Input: part model. Units: mm. Frame: model coordinates. Round coordinates to 2 decimals unless told otherwise and drop trailing zeros. Write each loop counter-clockwise with the first axis right and the second up, starting at its lowest first coordinate (ties: lowest second). Pieces come first, ordered by that corner, then holes. Notation, with made-up numbers: M -28,21 L 26,21 A20 ccw 26,28 Z; hole C 27,43 d11. An arc over 180 degrees is marked long. Answer as CSV lines item,"result". Start each with the question number.
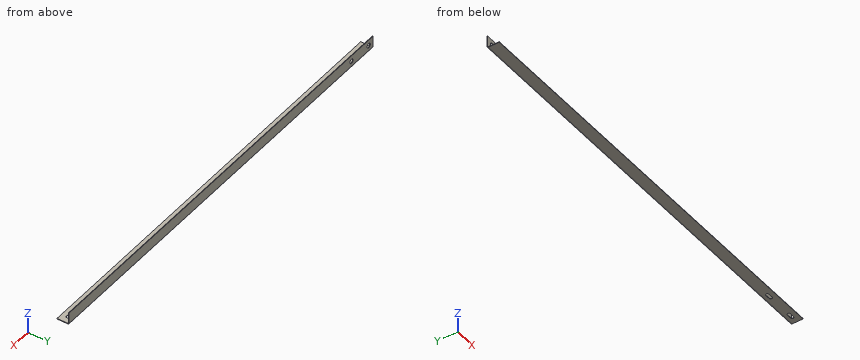
```python
from build123d import *

# Parameters (mm, degrees)
SKETCH1_W                    = 1415
SKETCH1_H                    = 40
BASE_FLANGE1_DEPTH           = 2
EDGE_FLANGE1_STRIP_W         = 13
EDGE_FLANGE1_STRIP_H         = 2
EDGE_FLANGE1_STRIP_CUT_DEPTH = 1415
EDGE_FLANGE1_DEPTH           = 1415
SKETCH9_R                    = 7.5
CUT_EXTRUDE1_DEPTH           = 920.516022359


# Sheet-metal steps are written as plain solids
with BuildPart() as part:
    # Sketch1 → Base-Flange1 (new body)
    with BuildSketch(Plane.XY):
        with Locations((-210.444287729, 62.85774027)):
            Rectangle(SKETCH1_W, SKETCH1_H)
        with BuildLine():
            Line((474.555712271, 57.85774027), (459.555712271, 57.85774027))
            ThreePointArc((459.555712271, 57.85774027), (454.555712271, 62.85774027), (459.555712271, 67.85774027))
            Line((459.555712271, 67.85774027), (474.555712271, 67.85774027))
            ThreePointArc((474.555712271, 67.85774027), (479.555712271, 62.85774027), (474.555712271, 57.85774027))
        make_face(mode=Mode.SUBTRACT)
        with BuildLine():
            Line((374.555712271, 57.85774027), (359.555712271, 57.85774027))
            ThreePointArc((359.555712271, 57.85774027), (354.555712271, 62.85774027), (359.555712271, 67.85774027))
            Line((359.555712271, 67.85774027), (374.555712271, 67.85774027))
            ThreePointArc((374.555712271, 67.85774027), (379.555712271, 62.85774027), (374.555712271, 57.85774027))
        make_face(mode=Mode.SUBTRACT)
    extrude(amount=-BASE_FLANGE1_DEPTH)

    # Edge-Flange1 strip (across the edge) → Edge-Flange1 strip cut (cut)
    with BuildSketch(Plane(origin=(497.055712271, 82.85774027, 0), x_dir=(0, -1, 0), z_dir=(-1, 0, 0))):
        with Locations((-2, -1)):
            Rectangle(EDGE_FLANGE1_STRIP_W, EDGE_FLANGE1_STRIP_H)
    extrude(amount=EDGE_FLANGE1_STRIP_CUT_DEPTH, mode=Mode.SUBTRACT)

    # Edge-Flange1 section (across the edge) → Edge-Flange1 (add)
    with BuildSketch(Plane(origin=(497.055712271, 82.85774027, 0), x_dir=(0, -1, 0), z_dir=(-1, 0, 0))):
        with BuildLine():
            Line((0, 2.5), (0, 38))
            Line((0, 38), (2, 38))
            Line((2, 38), (2, 2.5))
            ThreePointArc((2, 2.5), (2.732233047, 0.732233047), (4.5, 0))
            Line((4.5, 0), (4.5, -2))
            ThreePointArc((4.5, -2), (1.318019485, -0.681980515), (0, 2.5))
        make_face()
    extrude(amount=EDGE_FLANGE1_DEPTH)

    # Sketch9 → Cut-Extrude1 (cut, through all)
    with BuildSketch(Plane.XZ.offset(-80.85774027)):
        with Locations(Location((-897.944287729, 19, 0), (0, 0, 270))):
            Circle(SKETCH9_R)
        with Locations(Location((-817.944287729, 19, 0), (0, 0, 270))):
            Circle(SKETCH9_R)
    extrude(amount=-CUT_EXTRUDE1_DEPTH, mode=Mode.SUBTRACT)


solid = part.part
```
Item 1: Line query: line 1 (X direction, y = 82, z = 19); line 2 (Z direction, x = -140, y = 68.5); line 3 (Y direction, x = 409, z = 24). Output: solid intervals per line, ascending. Write a range as [from, to].
Item 2: Pin query (flat end, axial travel): pin 1 Ø4 at (x, y) = (-123, 57.5) entering from +Z; pin 2 Ø1 at (x, z) = (364.5, -1) entering from +Y; pin 3 Ø3 at (x, z) = (-132.5, 3) entering from -Y. Return the tip coordinate at first contact, or that it passes through.
Item 3: Cut plane C-C, the plane y = 50.5. Return loops of the section in (x, z).
Item 4: Cut plane B-B, the plane x = -367.5. Return loops of the section in (y, z).
Item 5: Cut plane A-A, the plane z = 19. Return loops of the section in (x, y).
Results list:
1,line 1,"[-917.94, -905.44], [-890.44, -825.44], [-810.44, 497.06]"
1,line 2,"[-2, 0]"
1,line 3,"[80.86, 82.86]"
2,pin 1,"z = 0"
2,pin 2,"y = 81.71"
2,pin 3,"y = 80.65"
3,outline,"M -917.94,-2 L 497.06,-2 L 497.06,0 L -917.94,0 Z"
4,outline,"M 42.86,-2 L 78.36,-2 A4.5 ccw 82.86,2.5 L 82.86,38 L 80.86,38 L 80.86,2.5 A2.5 cw 78.36,0 L 42.86,0 Z"
5,outline,"M -917.94,80.86 L -905.44,80.86 L -905.44,82.86 L -917.94,82.86 Z; M -890.44,80.86 L -825.44,80.86 L -825.44,82.86 L -890.44,82.86 Z; M -810.44,80.86 L 497.06,80.86 L 497.06,82.86 L -810.44,82.86 Z"
